For this review, use the dimensioned drawing (mm, ordinates from the lowest corner) and the shaded views. A direction names the side the tool comes from. Round coordinates to 2 decimals unless told otherwise and drop trailing zeros. Write each loop counter-clockwise with the first axis right and the second up, starting at its lowest first coordinate (ties: lowest second). Pieces come first, ordered by that corner, then holes. Notation, with made-up numbers: M 22.5,-31 L 26.5,-31 A22 cw 26.5,-12 Z; hole C -6.75,60.25 d1. An arc over 180 degrees is marked long. One line per question, with ' | ' between items. Start each with the question number.
Item 1: Machinability: for the marked faces 1 and 2, which of the approach directions +Z, -Z, +X, -X, +Y, -Y give a long, thin tool a straight path to every point of the face, cutting with its end or side? Answer none if there is none.
Item 2: Draft analysis for pull direction Y (two halves, no side actions). For the marked faces 3, 4, 5 and 6, state which applies: released by +Y, released by -Y, zero draft, split by the parting line, or undercut.
Item 3: Insertion check: pin 1 Ø3 at (x, z) = (32.5, 4.5) entering from -Y. The pin has a flat end and moves straight along its axis. Give the tip position at first contact, or say it passes through.
Item 4: Add section A-A, the plane z = 1.75. Give the number of separate pieces and of enclosed holes in the cut face, and give its area (3 significant figures).
Item 5: Add section D-D, the plane y = 6. State the section outline as (x, z) points, and give its area (3 significant figures).
Item 6: For L1, parallel to X at y = 17.5, z = 2.25; L2, parallel to X at y = 13.25, z = 4.25 (1 decimal); L3, parallel to X at y = 9.5, z = 2.25 (1 decimal), list the stretches that pass through material, from the lowest coordinate up.
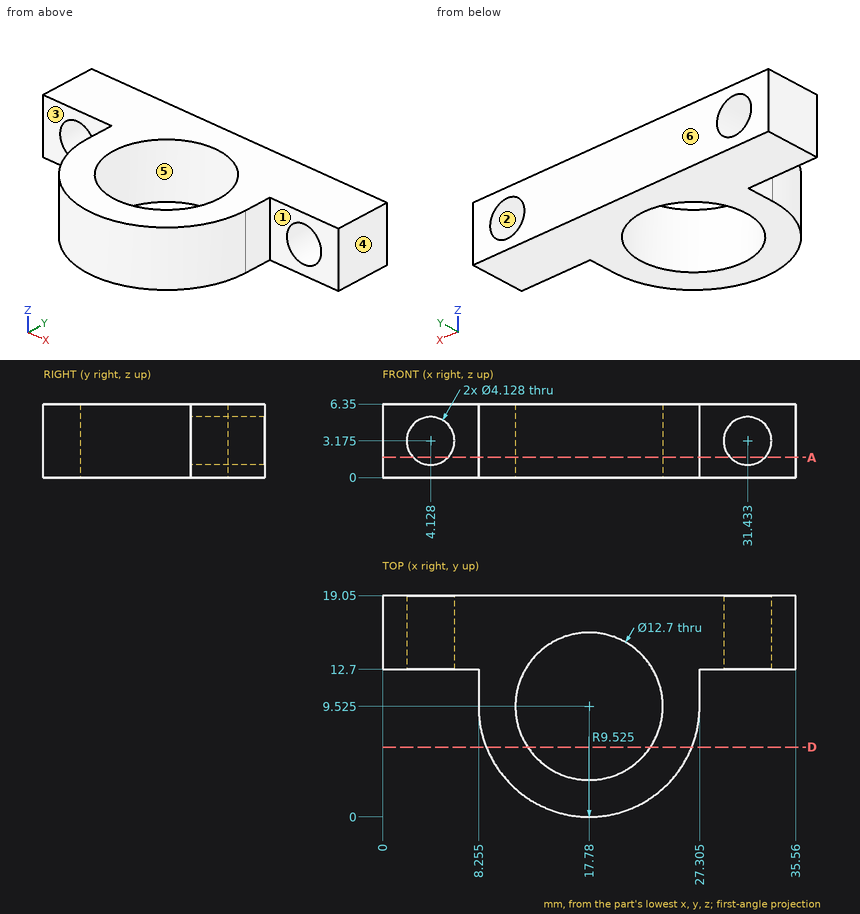
Computed values:
1) face 1: +Z, -Z, +X, -Y | face 2: +Y, -Y
2) face 3: released by -Y | face 4: zero draft | face 5: undercut | face 6: released by +Y
3) pin 1: stops at y = 12.7
4) separate pieces: 3 | enclosed holes: 1 | area: 264 mm^2
5) outline: M 8.93,0 L 12.5,0 L 12.5,6.35 L 8.93,6.35 Z; M 23.06,0 L 26.63,0 L 26.63,6.35 L 23.06,6.35 Z | area: 45.3 mm^2
6) L1: x = 0 to 2.28, 5.97 to 29.59, 33.28 to 35.56 | L2: x = 0 to 2.4, 5.9 to 12.6, 22.9 to 29.7, 33.2 to 35.6 | L3: x = 8.3 to 11.4, 24.1 to 27.3
